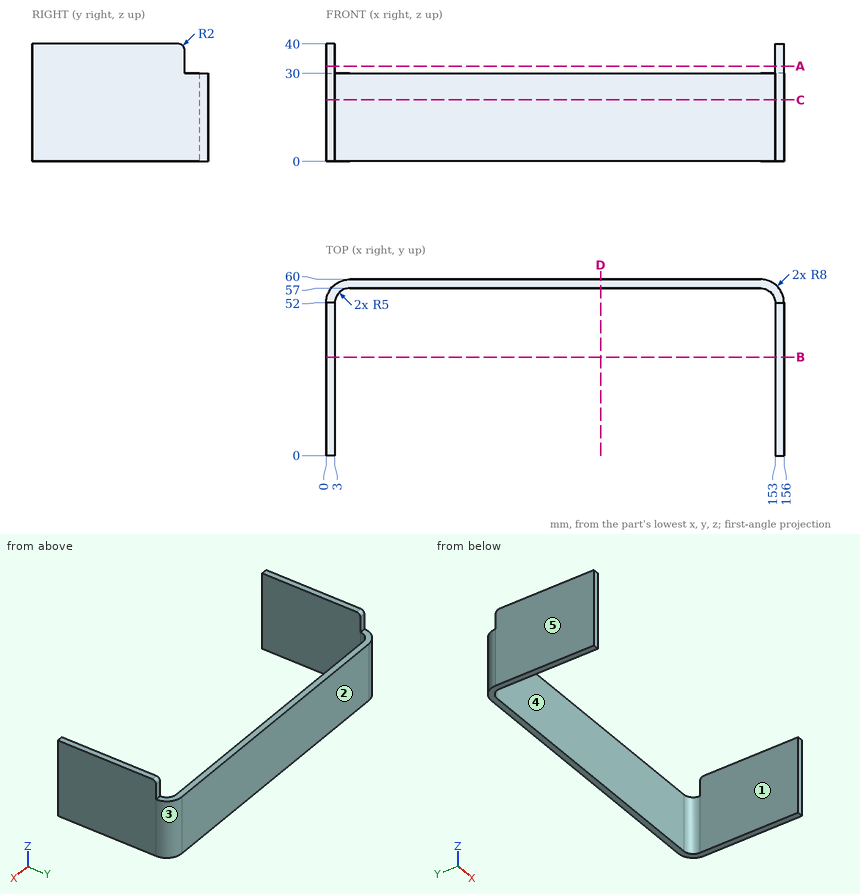
Geometry: see drawing. Coordinates: mm, zero at the bounding-box minimum. A direction names the side the tool comes from. Give positions to 0.01 mm unless a question says otherwise; leave off trailing zeros. Order: outer loops, then holes, each group sorted by start corner. A loop starts at its lowest first (then second) coordinate and runs counter-clockwise, first axis right, second up.
1. Draft query along X for the marked faces 3, 4 and 5. Return one class per face: released by +X, released by -X, zero draft, split by the parting line, or undercut.
Computed:
face 3: released by +X
face 4: undercut
face 5: released by -X
2. Set-up query: the marked faces 1 and 2. Return all of +Z, -Z, +X, -X, +Y, -Y with unobstructed straight access to the full face (end or side cutting, diameter ignored); none if empty.
Computed:
face 1: +Z, -Z, -Y
face 2: +Z, -Z, +X, -X, +Y
3. Cut plane A-A (z = 32.5). Return loops of the section in (x, y), and give its area (3 significant figures).
Computed:
outline: (0, 0) - (3, 0) - (3, 52) - (0, 52) - close; (153, 0) - (156, 0) - (156, 52) - (153, 52) - close
area: 312 mm2
4. Cut plane D-D (x = 93.5). Return loops of the section in (y, z), and give its area (3 significant figures).
Computed:
outline: (57, 0) - (60, 0) - (60, 30) - (57, 30) - close
area: 90.0 mm2
5. Cut plane B-B (y = 33.5). Return loops of the section in (x, z), and give its area (3 significant figures).
Computed:
outline: (0, 0) - (3, 0) - (3, 40) - (0, 40) - close; (153, 0) - (156, 0) - (156, 40) - (153, 40) - close
area: 240 mm2
6. Cut plane C-C (z = 21). Return loops of the section in (x, y).
Computed:
outline: (0, 0) - (3, 0) - (3, 52) arc R5 cw to (8, 57) - (148, 57) arc R5 cw to (153, 52) - (153, 0) - (156, 0) - (156, 52) arc R8 ccw to (148, 60) - (8, 60) arc R8 ccw to (0, 52) - close
7. Line query: probe 1 along X at (y, z) = (19, 9.5); probe 2 along Y at (x, z) = (18.5, 17); probe 3 along X at (y, z) = (54.5, 6). Output: solid intervals per line, ascending.
Computed:
probe 1: x = 0 to 3, 153 to 156
probe 2: y = 57 to 60
probe 3: x = 0.4 to 3.67, 152.33 to 155.6
8. Pin query (flat end, axial travel): pin 1 Ø3.5 at (x, z) = (1, 35.5) entering from +Y; pin 2 Ø4 at (x, y) = (86.5, 54.5) entering from +Z; pin 3 Ø12 at (x, z) = (42.5, 17.5) entering from -Y. Return the tip coordinate at first contact, or that it passes through.
Computed:
pin 1: stops at y = 52
pin 2: passes through
pin 3: stops at y = 57
